Source: CAD feature listing. Evaluate the final solid. Frame: model axes, mm. Give positions to 0.01 mm unless a question says otherwise; leave off trailing zeros. Order: outer loops, then holes, each group sorted by start corner. A loop starts at its lowest first (then second) coordinate and runs counter-clockwise, first axis right, second up.
from build123d import *

# Parameters (mm, degrees)
F1_DEPTH = 50
F2_R     = 4.99999


# Not quite as in the source:
# - a fillet or chamfer is up to 0.001 mm smaller than in the source, because OpenCascade refuses the exact size


with BuildPart() as f1:
    # F0 (on Front) → F1 (new body, symmetric)
    with BuildSketch(Plane.XZ):
        with BuildLine():
            Line((-50, 40), (-50, 0))
            Line((-50, 0), (0, 0))
            Line((0, 0), (50, 0))
            Line((50, 0), (50, 40))
            Line((50, 40), (35, 40))
            ThreePointArc((35, 40), (0, 5), (-35, 40))
            Line((-35, 40), (-50, 40))
        make_face()
    extrude(amount=F1_DEPTH, both=True)

    # F2 (radius 5 in the source; OpenCascade refuses exactly that, so slightly less here)
    f2_edges = [f1.edges().sort_by_distance(p)[0] for p in [
        (0, 50, 5),
    ]]
    fillet(f2_edges, radius=F2_R)


solid = f1.part
1) Section query B-B on y = -5. Output: boundary loops of the cut face in (x, z), and give its area (3 significant figures).
Checks:
outline: (-50, 0) - (50, 0) - (50, 40) - (35, 40) arc R35 cw to (-35, 40) - (-50, 40) - close
area: 2,080 mm2
2) First-contact query: pin 1 Ø1 at (x, y) = (17.5, 30) entering from -Z. Flat tip, straight axial feed; report the tip coordinate or a pass-through.
Checks:
pin 1: stops at z = 0
3) Ray query, L1, parallel to Z at x = 0, y = 37.5; L2, parallel to X at y = 4, z = 7.5; L3, parallel to X at y = -26, z = 38. Return the intervals inside material, ascending.
Checks:
L1: z = 0 to 5
L2: x = -50 to -12.99, 12.99 to 50
L3: x = -50 to -34.94, 34.94 to 50
